from build123d import *

# Parameters (mm, degrees)
SKETCH_1_W          = 100
SKETCH_1_H          = 80
SKETCH_1_R          = 10
EXTRUDE_1_DEPTH     = 78
CUT_EXTRUDE_1_REACH = 140.235
SKETCH_3_R          = 10


with BuildPart() as part:
    # Эскиз1 → Бобышка-Вытянуть1 (new body)
    with BuildSketch(Plane.XY):
        with Locations((0, 15)):
            Rectangle(SKETCH_1_W, SKETCH_1_H)
        with Locations((0, 15)):
            Circle(SKETCH_1_R, mode=Mode.SUBTRACT)
    extrude(amount=-EXTRUDE_1_DEPTH)

    # Эскиз3 → Вырез-Вытянуть1 (cut, up to next)
    with BuildSketch(Plane.ZY.offset(50), mode=Mode.PRIVATE) as cut_extrude_1_sk1:
        with Locations(Location((-39, -10, 0), (0, 0, 270))):
            Circle(SKETCH_3_R)
    cut_extrude_1_tool1 = extrude(cut_extrude_1_sk1.sketch, amount=-CUT_EXTRUDE_1_REACH, mode=Mode.PRIVATE) & part.part
    add(cut_extrude_1_tool1.solids().sort_by_distance((-50, -10, -39))[0], mode=Mode.SUBTRACT)


solid = part.part
Work out the finished part from the listing and answer in its coordinate system (mm). Coordinates: 2 decimals unless noted, no trailing zeros. Write each loop counter-clockwise with the first axis right and the second up, starting at its lowest first coordinate (ties: lowest second). Pieces come first, ordered by that corner, then holes. Notation, with made-up numbers: M -27.5,-35.75 L 13.5,-35.75 A18 ccw 13.5,-20.75 Z; hole C -25,8.25 d7. An arc over 180 degrees is marked long. Use one line per item in the form item = value. Start each with the question number.
1. The part is cut by section B-B (x = 0). Give the vertices of the cut face in (y, z).
2. The part is cut by section A-A (z = -39). Give the vertices of the cut face in (x, y), plus the area to 3 significant figures.
3. The part is cut by section C-C (y = -10). Give the vertices of the cut face in (x, z), plus the area to 3 significant figures.
4. Straight lines are drawn through the part: probe 1 along Z at (x, y) = (20.5, -10); probe 2 along Y at (x, z) = (0, -19); probe 3 along X at (y, z) = (9.5, -15.5). For each, find the intervals that lie inside material, in ascending order. Write a range as from..to.
5. The mould has two halves that part along Y. Classify faces 1 (the face through (-1, -25, -38)), 2 (the face through (-1.302, 24.915, -38.454)), 3 (the face through (-1, 55, -38)): released by +Y, released by -Y, zero draft, split by the parting line, or undercut.
6. The part is cut by section D-D (x = -20). Give the vertices of the cut face in (y, z).
Evaluation:
q1.outline = M -25,-78 L 5,-78 L 5,0 L -25,0 Z; M 25,-78 L 55,-78 L 55,0 L 25,0 Z; hole C -10,-39 d20
q2.outline = M -50,-25 L 50,-25 L 50,-20 L -50,-20 Z; M -50,0 L 50,0 L 50,55 L -50,55 Z; hole C 0,15 d20
q2.area = 5,690 mm^2
q3.outline = M -50,-78 L 50,-78 L 50,-49 L -50,-49 Z; M -50,-29 L 50,-29 L 50,0 L -50,0 Z
q3.area = 5,800 mm^2
q4.probe_1 = -78..-49, -29..0
q4.probe_2 = -25..5, 25..55
q4.probe_3 = -50..-8.35, 8.35..50
q5.face_1 = released by -Y
q5.face_2 = undercut
q5.face_3 = released by +Y
q6.outline = M -25,-78 L 55,-78 L 55,0 L -25,0 Z; hole C -10,-39 d20
